For this review, take the finished solid that the model builds, in its own axes (mm). A direction names the side the tool comes from. Give positions to 0.01 mm unless a question says otherwise; leave off trailing zeros. Order: outer loops, then holes, each group sorted by start corner. A loop starts at its lowest first (then second) coordinate and runs counter-clockwise, first axis right, second up. Notation, with made-up numbers: M 10,82 L 43,82 A27 cw 43,101 Z; hole C 32,-19.5 d6. An arc over 180 degrees is marked long. Answer as CSV lines item,"result". Start each with the question number.
1. We need section B-B, the plane x = 0. Give the boundary of the cut face in (y, z).
2. We need section A-A, the plane y = 20. Give the boundary of the cut face in (x, z).
3. Machinability: for faces 1 (the flat face through (22, 3.5, 1)), 2 (the flat face through (0, 14, 0)), which of the approach directions +Z, -Z, +X, -X, +Y, -Y give a long, thin tool a straight path to every point of the face, cutting with its end or side? Answer none if there is none.
4. Mouldability with a two-part tool opening along Y and no side actions: class faces 3 (the flat face through (-30, 0, 1)), 4 (the flat face through (20, -7, 1)), 5 (the flat face through (0, 30, 1)) as pulls with the +Y half, pulls with the -Y half, needs draft (parallel to the pull), parting line crosses it, or undercut.
5. For line 1 along Y through (x, z) = (0, 2); line 2 along X through (y, z) = (20, 1); line 3 along Y through (x, z) = (-4.5, 2.6), list the stretches that pass through material, from the lowest coordinate up.
6. We need section C-C, the plane z = 0.7. Give the boundary of the cut face in (x, y).
7. We need section D-D, the plane x = 18. Give the boundary of the cut face in (y, z).
Autodesk Inventor part; units mm, degrees
ref_plane "YZ Plane" through (0, 0, 0) normal (1, 0, 0) x (0, 1, 0)
ref_plane "XZ Plane" through (0, 0, 0) normal (0, 1, 0) x (-1, 0, 0)
ref_plane "XY Plane" through (0, 0, 0) normal (0, 0, 1) x (1, 0, 0)
sketch "Sketch1" plane through (0, 0, 0) normal (0, 0, 1) x (1, 0, 0)
  line L0 (-20, 10) -> (20, 10)
  line L1 (20, -10) -> (-20, -10)
  line L2 (-20, -10) -> (-20, 10)
  line L3 (-20, 10) -> (20, -10) construction
  line L4 (20, 10) -> (-20, -10) construction
  line L5 (-30, -30) -> (30, -30)
  line L6 (30, -30) -> (30, 30)
  line L7 (30, 30) -> (-30, 30)
  line L8 (-30, 30) -> (-30, -30)
  line L9 (-30, -30) -> (30, 30) construction
  line L10 (30, -30) -> (-30, 30) construction
  line L11 (0, 10) -> (0, 20)
  line L12 (0, -10) -> (0, -20)
  circle A0 centre (0, 20) radius 1.5
  circle A1 centre (0, -20) radius 1.5
  line L13 (20, -3.5) -> (23, -3.5)
  line L14 (23, -3.5) -> (23, 3.5)
  line L15 (23, 3.5) -> (20, 3.5)
  line L16 (20, 10) -> (20, 3.5)
  line L17 (20, -3.5) -> (20, -10)
  point P0 (0, 0)
  point P1 (20, 0)
  dimension "d0" = 40
  dimension "d1" = 20
  dimension "d2" = 60
  dimension "d3" = 60
  dimension "d4" = 10
  dimension "d5" = 10
  dimension "d6" = 3
  dimension "d7" = 3
  dimension "d11" = 7
extrude "Extrusion2" add sketch "Sketch1" along normal blind 3
properties part number "Servo Holder BOTTOM"
Result set:
1,outline,"M -30,0 L -21.5,0 L -21.5,3 L -30,3 Z; M -18.5,0 L -10,0 L -10,3 L -18.5,3 Z; M 10,0 L 18.5,0 L 18.5,3 L 10,3 Z; M 21.5,0 L 30,0 L 30,3 L 21.5,3 Z"
2,outline,"M -30,0 L -1.5,0 L -1.5,3 L -30,3 Z; M 1.5,0 L 30,0 L 30,3 L 1.5,3 Z"
3,face 1,"+Z, -Z"
3,face 2,"-Z, +X, -X, +Y, -Y"
4,face 3,"needs draft"
4,face 4,"undercut"
4,face 5,"pulls with the +Y half"
5,line 1,"-30 to -21.5, -18.5 to -10, 10 to 18.5, 21.5 to 30"
5,line 2,"-30 to -1.5, 1.5 to 30"
5,line 3,"-30 to -10, 10 to 30"
6,outline,"M -30,-30 L 30,-30 L 30,30 L -30,30 Z; hole M -20,-10 L 20,-10 L 20,-3.5 L 23,-3.5 L 23,3.5 L 20,3.5 L 20,10 L -20,10 Z; hole C 0,-20 d3; hole C 0,20 d3"
7,outline,"M -30,0 L -10,0 L -10,3 L -30,3 Z; M 10,0 L 30,0 L 30,3 L 10,3 Z"
